Design review of the part built by this model. Coordinates are the model's own, in mm. Give positions to 0.01 mm unless a question says otherwise; leave off trailing zeros. Order: outer loops, then holes, each group sorted by start corner. A loop starts at its lowest first (then second) coordinate and runs counter-clockwise, first axis right, second up.
```python
from build123d import *

# Parameters (mm, degrees)
F0_W     = 25.4
F0_H     = 3.175
F1_DEPTH = 3.175
F6_DEPTH = 3.176


# Not quite as in the source:
# - the program builds the solid bodies; features that only make, move or delete a surface that nothing else refers to are left out


with BuildPart() as f1:
    # F0 (on Top) → F1 (new body)
    with BuildSketch(Plane.XY):
        with BuildLine():
            Line((-120.0661680937, 14.7140049219), (-109.9481630411, 14.7140049219))
            ThreePointArc((-109.9481630411, 14.7140049219), (-114.7266583166, 21.2874831724), (-120.0661680937, 27.4140049219))
            Line((-120.0661680937, 27.4140049219), (-120.0661680937, 14.7140049219))
        make_face()
        with BuildLine():
            ThreePointArc((-109.9481630411, -86.8859950781), (-94.6661680937, -36.0859950781), (-109.9481630411, 14.7140049219))
            Line((-109.9481630411, 14.7140049219), (-120.0661680937, 14.7140049219))
            Line((-120.0661680937, 14.7140049219), (-120.0661680937, -86.8859950781))
            Line((-120.0661680937, -86.8859950781), (-109.9481630411, -86.8859950781))
        make_face()
        with Locations((32.3338319063, 13.1265049219)):
            Rectangle(F0_W, F0_H)
        with BuildLine():
            Line((-94.6661680937, -86.8859950781), (-109.9481630411, -86.8859950781))
            ThreePointArc((-109.9481630411, -86.8859950781), (-114.7266583166, -93.4594733286), (-120.0661680937, -99.5859950781))
            Line((-120.0661680937, -99.5859950781), (-94.6661680937, -99.5859950781))
            Line((-94.6661680937, -99.5859950781), (-94.6661680937, -86.8859950781))
        make_face()
        with BuildLine():
            Line((-89.0957787633, 14.7140049219), (-94.6661680937, 14.7140049219))
            Line((-94.6661680937, 14.7140049219), (-109.9481630411, 14.7140049219))
            ThreePointArc((-109.9481630411, 14.7140049219), (-94.6661680937, -36.0859950781), (-109.9481630411, -86.8859950781))
            Line((-109.9481630411, -86.8859950781), (-94.6661680937, -86.8859950781))
            Line((-94.6661680937, -86.8859950781), (19.6338319063, -86.8859950781))
            Line((19.6338319063, -86.8859950781), (19.6338319063, -83.7109950781))
            Line((19.6338319063, -83.7109950781), (45.0338319063, -83.7109950781))
            Line((45.0338319063, -83.7109950781), (45.0338319063, -86.8859950781))
            Line((45.0338319063, -86.8859950781), (57.7338319063, -86.8859950781))
            Line((57.7338319063, -86.8859950781), (57.7338319063, 14.7140049219))
            Line((57.7338319063, 14.7140049219), (45.0338319063, 14.7140049219))
            Line((45.0338319063, 14.7140049219), (45.0338319063, 11.5390049219))
            Line((45.0338319063, 11.5390049219), (19.6338319063, 11.5390049219))
            Line((19.6338319063, 11.5390049219), (19.6338319063, 14.7140049219))
            Line((19.6338319063, 14.7140049219), (-89.0957787633, 14.7140049219))
        make_face()
        with Locations((32.3338319063, -85.2984950781)):
            Rectangle(F0_W, F0_H)
        with BuildLine():
            ThreePointArc((-120.0661680937, -99.5859950781), (-114.7266583166, -93.4594733286), (-109.9481630411, -86.8859950781))
            Line((-109.9481630411, -86.8859950781), (-120.0661680937, -86.8859950781))
            Line((-120.0661680937, -86.8859950781), (-120.0661680937, -99.5859950781))
        make_face()
        with BuildLine():
            Line((-109.9481630411, 14.7140049219), (-94.6661680937, 14.7140049219))
            Line((-94.6661680937, 14.7140049219), (-94.6661680937, 27.4140049219))
            Line((-94.6661680937, 27.4140049219), (-120.0661680937, 27.4140049219))
            ThreePointArc((-120.0661680937, 27.4140049219), (-114.7266583166, 21.2874831724), (-109.9481630411, 14.7140049219))
        make_face()
    extrude(amount=F1_DEPTH)

    # F0 (on Top) → F6 (cut, through all)
    with BuildSketch(Plane.XY):
        with BuildLine():
            ThreePointArc((-109.9481630411, -86.8859950781), (-94.6661680937, -36.0859950781), (-109.9481630411, 14.7140049219))
            Line((-109.9481630411, 14.7140049219), (-120.0661680937, 14.7140049219))
            Line((-120.0661680937, 14.7140049219), (-120.0661680937, -86.8859950781))
            Line((-120.0661680937, -86.8859950781), (-109.9481630411, -86.8859950781))
        make_face()
        with BuildLine():
            Line((-120.0661680937, 14.7140049219), (-109.9481630411, 14.7140049219))
            ThreePointArc((-109.9481630411, 14.7140049219), (-114.7266583166, 21.2874831724), (-120.0661680937, 27.4140049219))
            Line((-120.0661680937, 27.4140049219), (-120.0661680937, 14.7140049219))
        make_face()
        with BuildLine():
            ThreePointArc((-120.0661680937, -99.5859950781), (-114.7266583166, -93.4594733286), (-109.9481630411, -86.8859950781))
            Line((-109.9481630411, -86.8859950781), (-120.0661680937, -86.8859950781))
            Line((-120.0661680937, -86.8859950781), (-120.0661680937, -99.5859950781))
        make_face()
    extrude(amount=F6_DEPTH, mode=Mode.SUBTRACT)


solid = f1.part
```
1. For pin 1 (1.6 mm diameter, centred on y = -93, z = 2, fed in from +X); pin 2 (1.5 mm diameter, centred on x = -71.5, z = 2.5, fed in from +Y); pin 3 (1.5 mm diameter, centred on x = 26.5, z = 1, fed in from -Y), all flat-tipped, find the tip position at first contact; note any pin that passes through.
Recorded:
pin 1: stops at x = -94.67
pin 2: stops at y = 14.71
pin 3: stops at y = -86.89
2. Take a section at A-A (z = 2). State the section outline as (x, y) points (3 decimals), then the cut area to 3 significant figures.
Recorded:
outline: (-120.066, -99.586) - (-94.666, -99.586) - (-94.666, -86.886) - (57.734, -86.886) - (57.734, 14.714) - (-94.666, 14.714) - (-94.666, 27.414) - (-120.066, 27.414) arc R92.075 cw to start
area: 16,500 mm2
3. Take a section at C-C (y = 16.5). State the section outline as (x, z) points (3 decimals).
Recorded:
outline: (-111.16, 0) - (-94.666, 0) - (-94.666, 3.175) - (-111.16, 3.175) - close
4. Take a section at B-B (x = -63.5). State the section outline as (y, z) points (3 decimals).
Recorded:
outline: (-86.886, 0) - (14.714, 0) - (14.714, 3.175) - (-86.886, 3.175) - close
5. For line 1 along Y through (x, z) = (-44, 0.45); line 2 along X through (y, z) = (-6.5, 2.05); line 3 along Y through (x, z) = (-102.5, 1.1), list the stretches that pass through material, from the lowest coordinate up.
Recorded:
line 1: y = -86.89 to 14.71
line 2: x = -99.55 to 57.73
line 3: y = -99.59 to -73.25, 1.08 to 27.41
